Check sheet for the modelled part. Datum: model origin and axes. Units: mm. Face numbers are marked on the shaded views. Give positions to 0.01 mm unless a question says otherwise; leave off trailing zeros. Write each loop counter-clockwise with the first axis right and the second up, starting at its lowest first coordinate (ties: lowest second). Pieces come first, ordered by that corner, then holes. Notation, with made-up numbers: (76.5, -1.5) -> (103.5, -1.5) arc R28 ccw to (103.5, 28.5) -> close; hole circle Ø9 at (44, 70.25). An arc over 180 degrees is marked (long way). Return JSON: item names as keys, results as strings.
from build123d import *

# Parameters (mm, degrees)
F0_W     = 63.5
F0_H     = 63.5
F1_DEPTH = 6.35
F2_R     = 12.7
F3_DEPTH = 6.35
F4_R     = 2.54
F5_DEPTH = 6.35


with BuildPart() as f1:
    # F0 (on Top) → F1 (new body)
    with BuildSketch(Plane.XY):
        Rectangle(F0_W, F0_H)
    extrude(amount=F1_DEPTH)

    # F2 (on Top) → F3 (cut, through all)
    with BuildSketch(Plane.XY):
        Circle(F2_R)
    extrude(amount=F3_DEPTH, mode=Mode.SUBTRACT)

    # F4 (on Top) → F5 (cut, through all)
    with BuildSketch(Plane.XY):
        with Locations((-26.67, 26.67)):
            Circle(F4_R)
    extrude(amount=F5_DEPTH, mode=Mode.SUBTRACT)


solid = f1.part
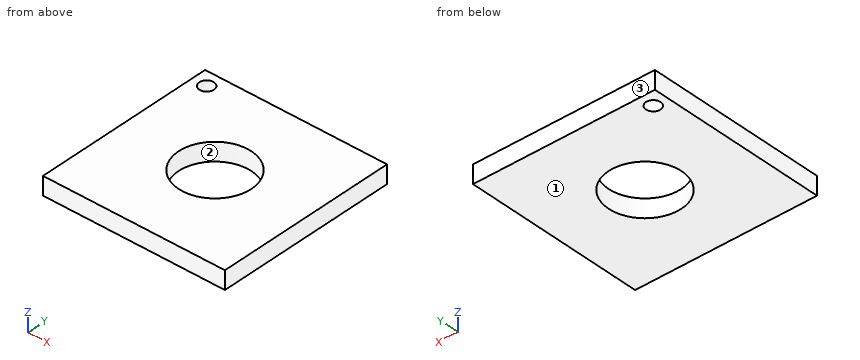
(1) Cross-section at C-C on z = 2.25. Enter the section's corners in (x, y), then the cut area to 3 significant figures.
Reply:
{"outline": "(-31.75, -31.75) -> (31.75, -31.75) -> (31.75, 31.75) -> (-31.75, 31.75) -> close; hole circle Ø5.08 at (-26.67, 26.67); hole circle Ø25.4 at (0, 0)", "area": "3,510 mm^2"}
(2) Thickness scan on L1, parallel to Y at x = -26.67, z = 1.75; L2, parallel to Y at x = 0, z = 2.25; L3, parallel to X at y = 25, z = 4.25. Record the ranges inside material, lowest first.
Reply:
{"L1": "-31.75 to 24.13, 29.21 to 31.75", "L2": "-31.75 to -12.7, 12.7 to 31.75", "L3": "-31.75 to -28.58, -24.76 to 31.75"}
(3) Cross-section at A-A on y = 0. Enter the section's corners in (x, z), then the cut area to 3 significant figures.
Reply:
{"outline": "(-31.75, 0) -> (-12.7, 0) -> (-12.7, 6.35) -> (-31.75, 6.35) -> close; (12.7, 0) -> (31.75, 0) -> (31.75, 6.35) -> (12.7, 6.35) -> close", "area": "242 mm^2"}
(4) Release check for a two-part mould opening along Y. For the marked faces 1, 2 and 3 record: pulls with the +Y half, pulls with the -Y half, needs draft (parallel to the pull), parting line crosses it, or undercut.
Reply:
{"face 1": "needs draft", "face 2": "undercut", "face 3": "pulls with the +Y half"}
(5) Cross-section at B-B on x = -26.67. Enter the section's corners in (y, z), then the cut area to 3 significant figures.
Reply:
{"outline": "(-31.75, 0) -> (24.13, 0) -> (24.13, 6.35) -> (-31.75, 6.35) -> close; (29.21, 0) -> (31.75, 0) -> (31.75, 6.35) -> (29.21, 6.35) -> close", "area": "371 mm^2"}
